Verification items for the finished model (mm, model axes). A direction names the side the tool comes from. Round coordinates to 2 decimals unless told otherwise and drop trailing zeros. Write item = value, one per line.
```python
from build123d import *

# Parameters (mm, degrees)
PAD011_DEPTH         = 3
PAD011_TAPER         = -5
PAD012_DEPTH         = 2.8
SKETCH036_R          = 1.5
HOLE001_DEPTH        = 2.2
SKETCH034_R          = 14.1
SKETCH047_R          = 14.1
SKETCH048_R          = 11.28
SKETCH028_R          = 3.5
POCKET010_DEPTH      = 16.001
SKETCH073_R          = 1.4
POCKET023_DEPTH      = 2.5
POCKET019_DEPTH      = 1.2
POCKET012_DEPTH      = 5
SKETCH072_W          = 35
SKETCH072_H          = 19.3
POCKET022_DEPTH      = 16.001
POCKET022_DEPTH_BACK = 0.001
SKETCH_W             = 37
SKETCH_H             = 5
PAD_DEPTH            = 7.5
SKETCH058_W          = 30.8
SKETCH058_H          = 2.1
POCKET_DEPTH         = 7
POCKET021_DEPTH      = 5.5


with BuildPart() as part:
    # Sketch024 → Pad011 (new body)
    with BuildSketch(Plane.XY):
        with BuildLine():
            Line((-45, 24), (-45, -24))
            ThreePointArc((-45, -24), (-44.414214, -25.414214), (-43, -26))
            Line((-43, -26), (43, -26))
            ThreePointArc((43, -26), (44.414214, -25.414214), (45, -24))
            Line((45, -24), (45, 24))
            ThreePointArc((45, 24), (44.414214, 25.414214), (43, 26))
            Line((43, 26), (-43, 26))
            ThreePointArc((-43, 26), (-44.414214, 25.414214), (-45, 24))
        make_face()
    extrude(amount=-PAD011_DEPTH, taper=PAD011_TAPER)

    # Sketch033 → Pad012 (join)
    with BuildSketch(Plane.XZ.offset(-22)):
        with BuildLine():
            Line((-39, 0), (39, 0))
            Line((39, 0), (39, -8))
            ThreePointArc((37, -10), (38.414214, -9.414214), (39, -8))
            Line((37, -10), (-37, -10))
            ThreePointArc((-39, -8), (-38.414214, -9.414214), (-37, -10))
            Line((-39, -8), (-39, 0))
        make_face()
    pad012 = extrude(amount=PAD012_DEPTH)

    # Sketch036 → Hole001 (cut)
    with BuildSketch(Plane.XZ.offset(-22)):
        with Locations((-35, -6.5)):
            Circle(SKETCH036_R)
        with Locations((35, -6.5)):
            Circle(SKETCH036_R)
    hole001 = extrude(amount=HOLE001_DEPTH, mode=Mode.SUBTRACT)

    # Mirrored: Pad012, Hole001 across XZ
    add(pad012.mirror(Plane.XZ))
    add(hole001.mirror(Plane.XZ), mode=Mode.SUBTRACT)

    # Sketch034 → AdditiveLoft section 0
    with BuildSketch(Plane.XY.offset(-3)):
        with Locations((10.5, 0)):
            Circle(SKETCH034_R)
    # Sketch047 → AdditiveLoft section 1
    with BuildSketch(Plane.XY.offset(-10.5)):
        with Locations((10.5, 0)):
            Circle(SKETCH047_R)
    # Sketch048 → AdditiveLoft section 2
    with BuildSketch(Plane.XY.offset(-16)):
        with Locations((10.5, 0)):
            Circle(SKETCH048_R)
    loft(ruled=True)

    # Sketch026 → Groove (revolve, cut)
    with BuildSketch(Plane(origin=(10.5, 0, 0), x_dir=(1, 0, 0), z_dir=(0, -1, 0))):
        with BuildLine():
            Line((0, 0), (12.7, 0))
            Line((12.7, 0), (12.7, -7))
            ThreePointArc((12.2, -7.5), (12.553553, -7.353553), (12.7, -7))
            Line((12.2, -7.5), (10.2, -7.5))
            Line((7.5, -13), (10.2, -7.5))
            Line((0, -13), (7.5, -13))
            Line((0, -13), (0, 0))
        make_face()
    revolve(axis=Axis((10.5, 0, 0), (0, 0, 1)), mode=Mode.SUBTRACT)

    # Sketch028 → Pocket010 (cut, through all)
    with BuildSketch(Plane.XY):
        with Locations((10.5, 0)):
            Circle(SKETCH028_R)
    extrude(amount=-POCKET010_DEPTH, mode=Mode.SUBTRACT)

    # Sketch073 → Pocket023 (cut)
    with BuildSketch(Plane.XY.offset(-16)):
        with Locations((10.5, -8)):
            Circle(SKETCH073_R)
        with Locations((10.5, 8)):
            Circle(SKETCH073_R)
    extrude(amount=POCKET023_DEPTH, mode=Mode.SUBTRACT)

    # Sketch053 → Pocket019 (cut)
    with BuildSketch(Plane.XY.offset(-3.5)):
        with BuildLine():
            Line((-42, 15.175), (-42, -18.925))
            ThreePointArc((-42, -18.925), (-41.941421, -19.066421), (-41.8, -19.125))
            Line((-41.8, -19.125), (-5.2, -19.125))
            ThreePointArc((-5.2, -19.125), (-5.058579, -19.066421), (-5, -18.925))
            Line((-5, -18.925), (-5, 15.175))
            ThreePointArc((-5, 15.175), (-5.058579, 15.316421), (-5.2, 15.375))
            Line((-5.2, 15.375), (-41.8, 15.375))
            ThreePointArc((-41.8, 15.375), (-41.941421, 15.316421), (-42, 15.175))
        make_face()
    extrude(amount=POCKET019_DEPTH, mode=Mode.SUBTRACT)

    # Sketch030 → Pocket012 (cut)
    with BuildSketch(Plane.XY.offset(-0.5)):
        Polygon((-30.5, 15.375), (-16.5, 15.375), (-16.5, 9.875), (-6, 9.875), (-6, -14.125), (-15, -14.125), (-15, -18.125), (-32, -18.125), (-32, -14.125), (-41, -14.125), (-41, 9.875), (-30.5, 9.875), align=None)
    extrude(amount=-POCKET012_DEPTH, mode=Mode.SUBTRACT)

    # Sketch072 → Pocket022 (cut, two sides)
    with BuildSketch(Plane.XY) as pocket022_sk:
        with Locations((-23.5, 0.025)):
            Rectangle(SKETCH072_W, SKETCH072_H)
    extrude(amount=-POCKET022_DEPTH, mode=Mode.SUBTRACT)
    extrude(pocket022_sk.sketch, amount=POCKET022_DEPTH_BACK, mode=Mode.SUBTRACT)

    # Sketch → Pad (join, symmetric)
    with BuildSketch(Plane.YZ.offset(33.5)):
        with Locations((0, -2.5)):
            Rectangle(SKETCH_W, SKETCH_H)
    extrude(amount=PAD_DEPTH, both=True)

    # Sketch058 → Pocket (cut, symmetric)
    with BuildSketch(Plane.YZ.offset(33.5)):
        with Locations((0, -1.05)):
            Rectangle(SKETCH058_W, SKETCH058_H)
    extrude(amount=POCKET_DEPTH, both=True, mode=Mode.SUBTRACT)

    # Sketch059 → Pocket021 (cut, symmetric)
    with BuildSketch(Plane.YZ.offset(33.5)):
        Polygon((-15.4, 0), (-15.4, -2.1), (-14.5, -2.1), (-14.5, -22.1), (14.5, -22.1), (14.5, -2.1), (15.4, -2.1), (15.4, 0), align=None)
    extrude(amount=POCKET021_DEPTH, both=True, mode=Mode.SUBTRACT)


solid = part.part
```
(1) Go/stop test with flat-tipped pins: pin 1 Ø4 at (x, z) = (29.5, -8) entering from +Y; pin 2 Ø1.2 at (y, z) = (-4, -1) entering from -X; pin 3 Ø1.4 at (y, z) = (-20, -6.5) entering from +X. Record where each tip stops, or that it passes through.
Filled sheet:
pin_1 = 22
pin_2 = -45.14
pin_3 = 39
(2) Set-up check for faces 4 (the face through (-11, 9.875, -1)), 5 (the face through (1, -21, -10)), 6 (the face through (1, -19.2, -6)), 7 (the face through (16, -9, -7.5)): record each of +Z, -Z, +X, -X, +Y, -Y from which the full face is reachable in a straight line by a thin tool's end or side.
Filled sheet:
face_4 = -Z
face_5 = -Z, +X, -X, -Y
face_6 = -Z, +X, -X
face_7 = +Z
(3) Material ranges on probe 1 along Y at (x, z) = (10.5, -5); probe 2 along Z at (x, y) = (35, 21); probe 3 along Y at (x, z) = (9.5, -9.5), recorded low to high. Write a range as from..to.
Filled sheet:
probe_1 = -22..-19.2, -14.1..-12.7, 12.7..14.1, 19.2..22
probe_2 = -10..-8, -5..0
probe_3 = -22..-19.2, -14.06..-9.16, 9.16..14.06, 19.2..22
(4) Sectioned sample at A-A, the plane y = 0. Count the separate pieces of the cut face and the enclosed holes in it, and give its area (3 significant figures).
Filled sheet:
separate_pieces = 4
enclosed_holes = 0
area = 175 mm2
(5) Draft check along Z on faces 1 (the face through (33.8, 20.9, -7.4)), 2 (the face through (10, -8, -13.5)), 3 (the face through (34, 14.5, -4)). Enter one of: released by +Z, released by -Z, zero draft, split by the parting line, or undercut.
Filled sheet:
face_1 = undercut
face_2 = released by -Z
face_3 = zero draft
